Geometry: see drawing. Coordinates: mm, zero at the bounding-box minimum. A direction names the side the tool comes from. Coordinates: 2 decimals unless noted, no trailing zeros. Write each loop counter-clockwise with the first axis right and the second up, starting at its lowest first coordinate (ties: lowest second). Pieces come first, ordered by that corner, then holes.
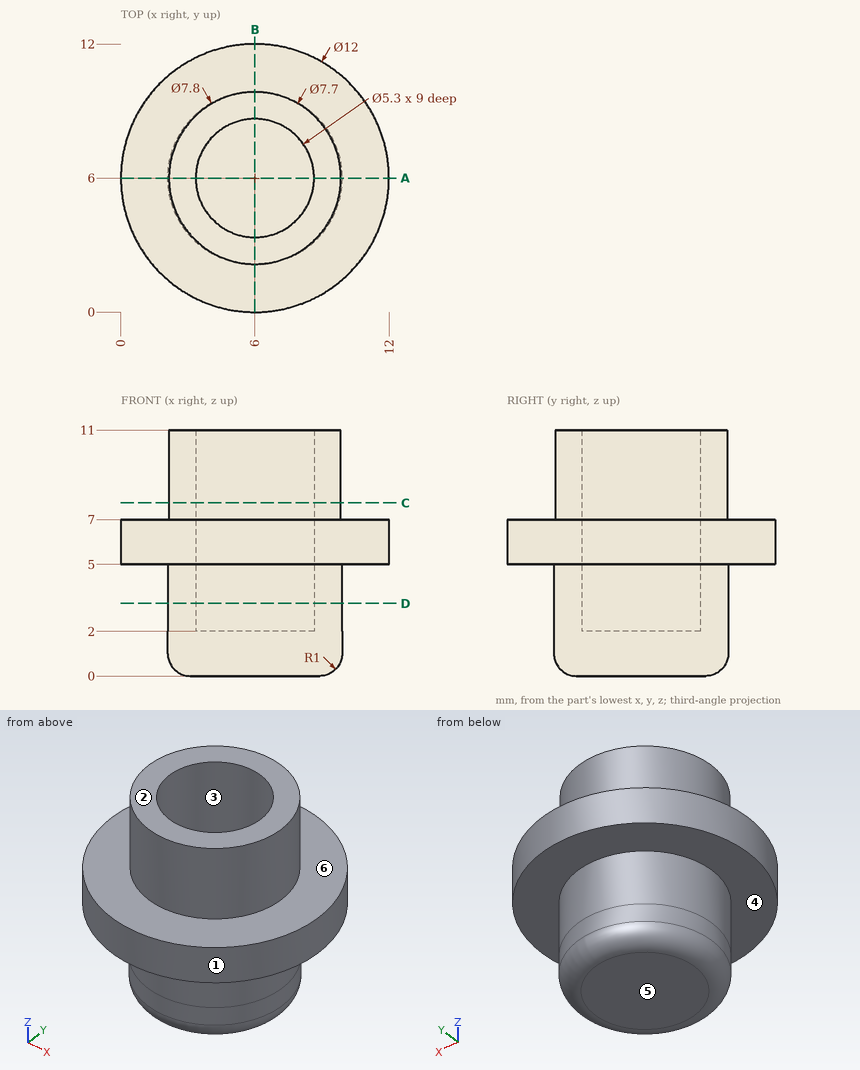
Item 1: Pin query (flat end, axial travel): pin 1 (3 mm diameter, centred on x = 4, y = 7.5, fed in from -Z); pin 2 (2 mm diameter, centred on y = 3, z = 1.5, fed in from -X); pin 3 (4 mm diameter, centred on y = 3.5, z = 9.5, fed in from -X); pin 4 (3 mm diameter, centred on y = 8, z = 3, fed in from -X). Return the tip coordinate at first contact, or that it passes through.
Derived:
pin 1: stops at z = 0
pin 2: stops at x = 2.65
pin 3: stops at x = 2.18
pin 4: stops at x = 2.13
Item 2: Set-up query: the marked faces 4, 5 and 6. Return all of +Z, -Z, +X, -X, +Y, -Y with unobstructed straight access to the full face (end or side cutting, diameter ignored); none if empty.
Derived:
face 4: -Z
face 5: -Z, +X, -X, +Y, -Y
face 6: +Z
Item 3: Section D-D, the plane z = 3.25. Output: boundary loops of the cut face in (x, y).
Derived:
outline: circle Ø7.8 at (6, 6); hole circle Ø5.3 at (6, 6)
Item 4: Material intervals for probe 1 along Y at (x, z) = (6, 6); probe 2 along Y at (x, z) = (6, 8); probe 3 along X at (y, z) = (7.75, 5.5), sorted ascending.
Derived:
probe 1: y = 0 to 3.35, 8.65 to 12
probe 2: y = 2.15 to 3.35, 8.65 to 9.85
probe 3: x = 0.26 to 4.01, 7.99 to 11.74
Item 5: Pull-direction query (X, two-part tool) for the marked faces 1, 2 and 3; classes: released by +X, released by -X, zero draft, split by the parting line, or undercut.
Derived:
face 1: split by the parting line
face 2: zero draft
face 3: undercut
Item 6: Section C-C, the plane z = 7.75. Output: boundary loops of the cut face in (x, y).
Derived:
outline: circle Ø7.7 at (6, 6); hole circle Ø5.3 at (6, 6)
Item 7: Section A-A, the plane y = 6. Output: boundary loops of the cut face in (x, z).
Derived:
outline: (0, 5) - (2.1, 5) - (2.1, 1) arc R1 ccw to (3.1, 0) - (8.9, 0) arc R1 ccw to (9.9, 1) - (9.9, 5) - (12, 5) - (12, 7) - (9.85, 7) - (9.85, 11) - (8.65, 11) - (8.65, 2) - (3.35, 2) - (3.35, 11) - (2.15, 11) - (2.15, 7) - (0, 7) - close
